Could you check a few things on this model? Use its own coordinates, in mm. Give positions to 0.01 mm unless a question says otherwise; leave off trailing zeros. Loops run counter-clockwise (first coordinate to the right, second up) from the corner with the lowest first, then second, coordinate; pieces in that order, holes last. Notation, with made-up numbers: M -8.5,-1 L 48.5,-1 A32 ccw 48.5,30 Z; hole C 59.5,76.5 d1. An arc over 180 degrees is marked long. Use CSV: the item, a comma, the result in double quotes.
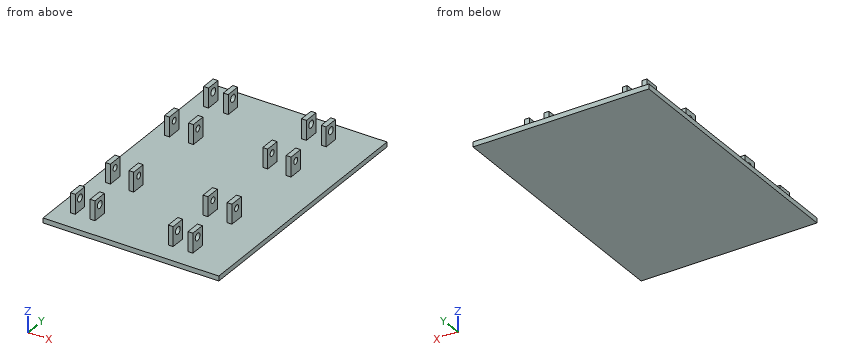
```python
from build123d import *

# Parameters (mm, degrees)
SKETCH1_W               = 228.6
SKETCH1_H               = 339.725
BOSS_EXTRUDE1_DEPTH     = 6.35
SKETCH2_W               = 6.35
SKETCH2_H               = 19.05
BOSS_EXTRUDE2_DEPTH     = 25.4
SKETCH3_R               = 4.7625
SKETCH3_R_2             = 4
CUT_EXTRUDE1_DEPTH      = 20.05
CUT_EXTRUDE1_DEPTH_BACK = 210.55


with BuildPart() as part:
    # Sketch1 → Boss-Extrude1 (new body)
    with BuildSketch(Plane.XY):
        with Locations((114.3, -169.8625)):
            Rectangle(SKETCH1_W, SKETCH1_H)
    extrude(amount=BOSS_EXTRUDE1_DEPTH)

    # Sketch2 → Boss-Extrude2 (add)
    with BuildSketch(Plane.XY.offset(6.35)):
        with Locations((22.225, -35.2425)):
            Rectangle(SKETCH2_W, SKETCH2_H)
        with Locations((47.879, -35.2425)):
            Rectangle(SKETCH2_W, SKETCH2_H)
        with Locations((149.479, -35.2425)):
            Rectangle(SKETCH2_W, SKETCH2_H)
        with Locations((175.133, -35.2425)):
            Rectangle(SKETCH2_W, SKETCH2_H)
        with Locations((22.225, -304.4825)):
            Rectangle(SKETCH2_W, SKETCH2_H)
        with Locations((47.879, -304.4825)):
            Rectangle(SKETCH2_W, SKETCH2_H)
        with Locations((149.479, -304.4825)):
            Rectangle(SKETCH2_W, SKETCH2_H)
        with Locations((175.133, -304.4825)):
            Rectangle(SKETCH2_W, SKETCH2_H)
        with Locations((19.685, -110.1598)):
            Rectangle(SKETCH2_W, SKETCH2_H)
        with Locations((50.419, -109.5248)):
            Rectangle(SKETCH2_W, SKETCH2_H)
        with Locations((146.939, -109.5248)):
            Rectangle(SKETCH2_W, SKETCH2_H)
        with Locations((177.673, -110.1598)):
            Rectangle(SKETCH2_W, SKETCH2_H)
        with Locations((177.673, -229.5652)):
            Rectangle(SKETCH2_W, SKETCH2_H)
        with Locations((146.939, -230.2002)):
            Rectangle(SKETCH2_W, SKETCH2_H)
        with Locations((50.419, -230.2002)):
            Rectangle(SKETCH2_W, SKETCH2_H)
        with Locations((19.685, -229.5652)):
            Rectangle(SKETCH2_W, SKETCH2_H)
    extrude(amount=BOSS_EXTRUDE2_DEPTH)

    # Sketch3 → Cut-Extrude1 (cut, two sides)
    with BuildSketch(Plane.ZY.offset(-19.05)) as cut_extrude1_sk:
        with Locations((22.225, -35.2425)):
            Circle(SKETCH3_R)
        with Locations((22.225, -229.5652)):
            Circle(SKETCH3_R_2)
        with Locations((22.225, -304.4825)):
            Circle(SKETCH3_R)
        with Locations((22.225, -110.1598)):
            Circle(SKETCH3_R_2)
    extrude(amount=CUT_EXTRUDE1_DEPTH, mode=Mode.SUBTRACT)
    extrude(cut_extrude1_sk.sketch, amount=-CUT_EXTRUDE1_DEPTH_BACK, mode=Mode.SUBTRACT)


solid = part.part
```
1. Please list where these lines run through material, in increasing order: line 1 (X direction, y = -44, z = 27.5); line 2 (X direction, y = -221.5, z = 9.5); line 3 (Z direction, x = 88.5, y = -91).
Outcome:
line 1,"19.05 to 25.4, 44.7 to 51.05, 146.3 to 152.65, 171.96 to 178.31"
line 2,"16.51 to 22.86, 47.24 to 53.59, 143.76 to 150.11, 174.5 to 180.85"
line 3,"0 to 6.35"
2. I want a section at B-B, the plane x = 132. List the corners of the cut face in (y, z) for me (3 decimals), then the cut area to 3 significant figures.
Outcome:
outline,"M -339.725,0 L 0,0 L 0,6.35 L -339.725,6.35 Z"
area,"2,160 mm2"
3. I want a section at A-A, the plane z = 12. Give the number of separate pieces and of enclosed holes in the cut face, then the cut area to 3 significant figures.
Outcome:
separate pieces,"16"
enclosed holes,"0"
area,"1,940 mm2"
4. I'm going to push flat-ended pins straight in: pin 1 Ø7 at (x, z) = (23, 13.5) entering from -Y; pin 2 Ø6 at (x, y) = (66, -46) entering from +Z; pin 3 Ø9.5 at (y, z) = (-35, 17.5) entering from -X. Where does each tip first touch, or does it pass through?
Outcome:
pin 1,"y = -314.01"
pin 2,"z = 6.35"
pin 3,"x = 19.05"
5. I want a section at C-C, the plane y = -198.5. List the corners of the cut face in (x, z) for me.
Outcome:
outline,"M 0,0 L 228.6,0 L 228.6,6.35 L 0,6.35 Z"
